For this review, use the dimensioned drawing (mm, ordinates from the lowest corner) and the shaded views. A direction names the side the tool comes from. Round coordinates to 2 decimals unless told otherwise and drop trailing zeros. Order: outer loops, then holes, each group sorted by start corner. A loop starts at its lowest first (then second) coordinate and runs counter-clockwise, first axis right, second up. Notation, with made-up numbers: (-6, 44.5) - (6, 44.5) arc R32 ccw to (6, 82.5) - close; hole circle Ø6 at (57.5, 58). An arc over 180 degrees is marked (long way). Write item = value, one per line.
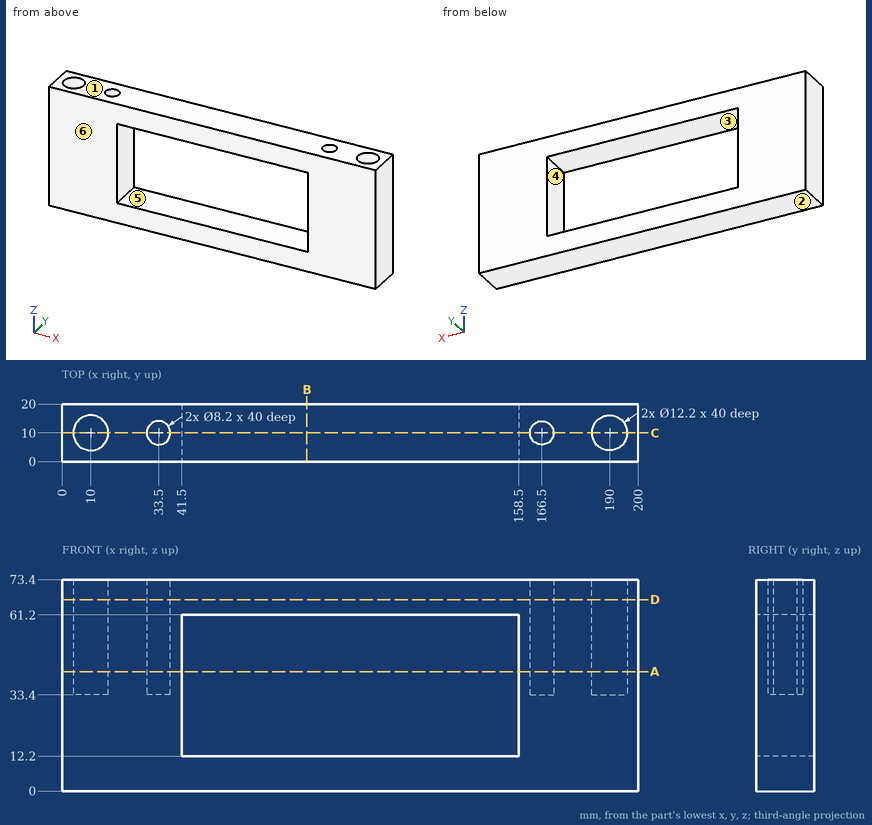
Item 1: Take a section at A-A, the plane z = 41.5. State the section outline as (x, y) points.
Data:
outline = (0, 0) - (41.5, 0) - (41.5, 20) - (0, 20) - close; (158.5, 0) - (200, 0) - (200, 20) - (158.5, 20) - close; hole circle Ø12.2 at (10, 10); hole circle Ø8.2 at (33.5, 10); hole circle Ø8.2 at (166.5, 10); hole circle Ø12.2 at (190, 10)
Item 2: The part is to be moulded in two halves that separate along Z. For the marked faces 1, 2, 3 and 4, say which applies: +Z half, -Z half, draft (parallel to the pull), parting line (faces both ways), or undercut.
Data:
face_1 = +Z half
face_2 = -Z half
face_3 = undercut
face_4 = undercut
Item 3: Insertion check: P1, Ø3.5, axis at x = 10, y = 11, coming from the +Z side. The pin has a flat end and moves straight along its axis. Give the tip position at first contact, or say it passes through.
Data:
P1 = 33.4
Item 4: Take a section at C-C, the plane y = 10. State the section outline as (x, z) points.
Data:
outline = (0, 0) - (200, 0) - (200, 73.4) - (196.1, 73.4) - (196.1, 33.4) - (183.9, 33.4) - (183.9, 73.4) - (170.6, 73.4) - (170.6, 33.4) - (162.4, 33.4) - (162.4, 73.4) - (37.6, 73.4) - (37.6, 33.4) - (29.4, 33.4) - (29.4, 73.4) - (16.1, 73.4) - (16.1, 33.4) - (3.9, 33.4) - (3.9, 73.4) - (0, 73.4) - close; hole (41.5, 12.2) - (158.5, 12.2) - (158.5, 61.2) - (41.5, 61.2) - close
Item 5: Take a section at D-D, the plane z = 66.5. State the section outline as (x, y) points, and give its area (3 significant figures).
Data:
outline = (0, 0) - (200, 0) - (200, 20) - (0, 20) - close; hole circle Ø12.2 at (10, 10); hole circle Ø8.2 at (33.5, 10); hole circle Ø8.2 at (166.5, 10); hole circle Ø12.2 at (190, 10)
area = 3,660 mm2
Item 6: For line 1 along Z through (x, y) = (90, 18.5); line 2 along Y through (x, z) = (166.5, 64); line 3 along X through (y, z) = (18.5, 55), list the stretches that pass through material, from the lowest coordinate up. Write a range as [from, to].
Data:
line_1 = [0, 12.2], [61.2, 73.4]
line_2 = [0, 5.9], [14.1, 20]
line_3 = [0, 41.5], [158.5, 200]
Item 7: Take a section at B-B, the plane x = 85. State the section outline as (y, z) points, and give its area (3 significant figures).
Data:
outline = (0, 0) - (20, 0) - (20, 12.2) - (0, 12.2) - close; (0, 61.2) - (20, 61.2) - (20, 73.4) - (0, 73.4) - close
area = 488 mm2
Item 8: For the marked faces 5 and 6, list the 3-axis set-ups (+Z, -Z, +X, -X, +Y, -Y) from which the entire face can be reached by the end or side of a thin tool; tool diameter is ignored.
Data:
face_5 = +Y, -Y
face_6 = +Z, -Z, +X, -X, -Y
